from build123d import *

# Parameters (mm, degrees)
SKETCH1_W           = 172.974
SKETCH1_H           = 102.108
BOSS_EXTRUDE1_DEPTH = 13.97
SKETCH2_R           = 7.4676
SKETCH2_R_2         = 3.014975044
SKETCH2_W           = 7.81218406
SKETCH2_H           = 2.407827673
BOSS_EXTRUDE3_DEPTH = 3.048
SKETCH3_R           = 7.4676
SKETCH3_R_2         = 3.014975044
BOSS_EXTRUDE5_DEPTH = 3.048


with BuildPart() as part:
    # Sketch1 → Boss-Extrude1 (new body)
    with BuildSketch(Plane.XY):
        with Locations((58.9637029, 33.169946412)):
            Rectangle(SKETCH1_W, SKETCH1_H)
        with BuildLine():
            Line((-27.5232971, 84.223946412), (-43.0172971, 84.223946412))
            ThreePointArc((-43.0172971, 84.223946412), (-57.385706894, 78.272356205), (-63.3372971, 63.903946412))
            Line((-63.3372971, 63.903946412), (-63.3372971, 2.435946412))
            ThreePointArc((-63.3372971, 2.435946412), (-57.385706894, -11.932463382), (-43.0172971, -17.884053588))
            Line((-43.0172971, -17.884053588), (-27.5232971, -17.884053588))
            Line((-27.5232971, -17.884053588), (-27.5232971, 84.223946412))
        make_face()
        with BuildLine():
            Line((160.9447029, 84.223946412), (145.4507029, 84.223946412))
            Line((145.4507029, 84.223946412), (145.4507029, -17.884053588))
            Line((145.4507029, -17.884053588), (160.9447029, -17.884053588))
            ThreePointArc((160.9447029, -17.884053588), (175.313112694, -11.932463382), (181.2647029, 2.435946412))
            Line((181.2647029, 2.435946412), (181.2647029, 63.903946412))
            ThreePointArc((181.2647029, 63.903946412), (175.313112694, 78.272356205), (160.9447029, 84.223946412))
        make_face()
    extrude(amount=BOSS_EXTRUDE1_DEPTH)

    # Sketch2 → Boss-Extrude3 (add)
    with BuildSketch(Plane(origin=(0, 0, 0), x_dir=(-1, 0, 0), z_dir=(0, 0, -1))):
        with Locations(Location((-163.4847029, 58.823946412, 0), (0, 0, 180))):
            Circle(SKETCH2_R)
        with Locations(Location((-170.337090886, 26.676001086, 0), (0, 0, 180))):
            Circle(SKETCH2_R_2)
        with Locations(Location((-163.221177768, 32.823656386, 0), (0, 0, 180))):
            Circle(SKETCH2_R_2)
        with Locations(Location((-156.732358191, 26.205188985, 0), (0, 0, 180))):
            Circle(SKETCH2_R_2)
        with Locations(Location((-163.721455714, 19.973644896, 0), (0, 0, 180))):
            Circle(SKETCH2_R_2)
        with Locations((-152.730393721, 74.856056835)):
            Rectangle(SKETCH2_W, SKETCH2_H)
    extrude(amount=BOSS_EXTRUDE3_DEPTH)

    # Sketch3 → Boss-Extrude5 (add)
    with BuildSketch(Plane(origin=(0, 0, 0), x_dir=(-1, 0, 0), z_dir=(0, 0, -1))):
        with Locations(Location((45.487523866, 28.516423037, 0), (0, 0, 180))):
            Circle(SKETCH3_R)
        with Locations(Location((44.957454366, 53.116068624, 0), (0, 0, 180))):
            Circle(SKETCH3_R_2)
        with Locations(Location((38.341819194, 59.818424813, 0), (0, 0, 180))):
            Circle(SKETCH3_R_2)
        with Locations(Location((45.457732312, 65.966080113, 0), (0, 0, 180))):
            Circle(SKETCH3_R_2)
        with Locations(Location((51.94655189, 59.347612713, 0), (0, 0, 180))):
            Circle(SKETCH3_R_2)
        Polygon((38.47340824, 76.391412748), (41.190295926, 76.391412748), (41.190295926, 73.983585075), (38.47340824, 73.983585075), (38.47340824, 71.443585075), (35.93340824, 71.443585075), (35.93340824, 73.983585075), (33.570295926, 73.983585075), (33.570295926, 76.391412748), (35.93340824, 76.391412748), (35.93340824, 78.931412748), (38.47340824, 78.931412748), align=None)
    extrude(amount=BOSS_EXTRUDE5_DEPTH)


solid = part.part
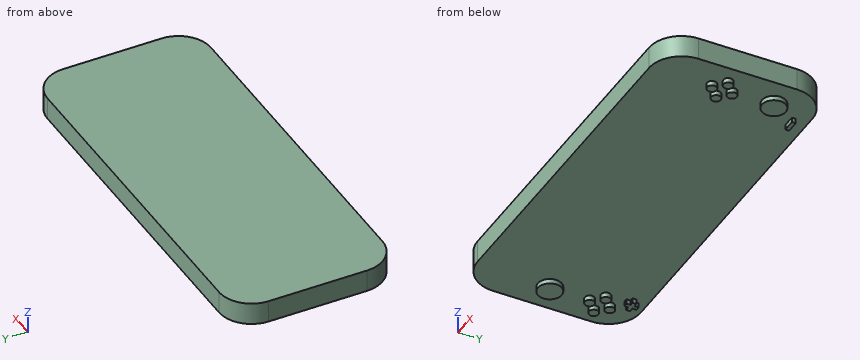
Could you check a few things on this model? Use its own coordinates, in mm. Round coordinates to 2 decimals unless told otherwise and drop trailing zeros. Order: outer loops, then holes, each group sorted by start corner. A loop starts at its lowest first (then second) coordinate and runs counter-clockwise, first axis right, second up. Notation, with made-up numbers: M 31,-24 L 36,-24 A20 cw 36,-8 Z; hole C 13,84.25 d6. An arc over 180 degrees is marked long. One line per item, written item: value.
(1) I'm going to push flat-ended pins straight in: P1, Ø2.5, axis at y = 74.5, z = -1, coming from the +X side; P2, Ø0.7, axis at y = 75, z = -1, coming from the -X side; P3, Ø2.5, axis at x = 153.5, z = -1.5, coming from the +Y side. Where does each tip first touch, or does it pass through?
Ans:
P1: stops at x = 178.72
P2: stops at x = -41.19
P3: stops at y = 76.06
(2) Imagine slicing it at B-B (y = 7). Write out the boundary of the cut face in (x, z), and give its area (3 significant figures).
Ans:
outline: M -63.34,0 L 181.26,0 L 181.26,13.97 L -63.34,13.97 Z
area: 3,420 mm^2
(3) I need wall thicknesses on line 1 along Z through (x, y) = (129, 44.5); line 2 along Y through (x, z) = (159, -0.75); line 3 along X through (y, z) = (64.5, -0.75). Which ranges of each line are inside material? Lowest first, please. Write a range as from..to.
Ans:
line 1: z = 0..13.97
line 2: y = 24.22..28.19, 52.85..64.79
line 3: x = -48.09..-42.82, 158.63..168.34
(4) Imagine slicing it at A-A (x = 58.5). Write out the boundary of the cut face in (y, z), and give its area (3 significant figures).
Ans:
outline: M -17.88,0 L 84.22,0 L 84.22,13.97 L -17.88,13.97 Z
area: 1,430 mm^2
